Check sheet for the modelled part. Datum: model origin and axes. Units: mm. Face numbers are marked on the shaded views. A direction names the side the tool comes from. Round coordinates to 2 decimals unless told otherwise and drop trailing zeros. Write each loop counter-clockwise with the first axis right and the second up, starting at its lowest first coordinate (ties: lowest second). Pieces come first, ordered by that corner, then holes. Notation, with made-up numbers: (32, 25) -> (49, 25) arc R21 cw to (49, 45) -> close; hole circle Ø7 at (66, -24.5). An arc over 180 degrees is marked (long way). One line per item, written item: value.
from build123d import *

# Parameters (mm, degrees)
SKETCH_1_W          = 30
SKETCH_1_H          = 3
EXTRUDE_1_DEPTH     = 45
SKETCH_1_3_W        = 7
SKETCH_1_3_H        = 20
SKETCH_1_3_W_2      = 30
SKETCH_1_3_H_2      = 3
EXTRUDE_2_DEPTH     = 3
SKETCH_2_W          = 55
SKETCH_2_H          = 40
EXTRUDE_3_DEPTH     = 2
SKETCH_3_W          = 30
SKETCH_3_H          = 2
EXTRUDE_4_DEPTH     = 5
SKETCH_4_W          = 30
SKETCH_4_H          = 15
CUT_EXTRUDE_1_DEPTH = 58.203583804
CUT_EXTRUDE_2_REACH = 60.824
SKETCH_6_R          = 1.6
FILLET_1_R          = 3
FILLET_2_R          = 3
CHAMFER_1_SIZE      = 3
CHAMFER_2_SIZE      = 1
FILLET_4_R          = 3


# Some blends are built 0.0001 mm under size
with BuildPart() as part:
    # 草图1 → 凸台-拉伸1 (new body)
    with BuildSketch(Plane(origin=(0, 0, 0), x_dir=(1, 0, 0), z_dir=(0, 1, 0))):
        Polygon((18, 10), (15, 10), (15, 7), (15, -10), (18, -10), align=None)
        with Locations((0, 8.5)):
            Rectangle(SKETCH_1_W, SKETCH_1_H)
        Polygon((-15, 7), (-15, 10), (-18, 10), (-18, -10), (-15, -10), align=None)
    extrude(amount=-EXTRUDE_1_DEPTH)

    # 草图1<3> → 凸台-拉伸2 (add)
    with BuildSketch(Plane(origin=(0, 0, 0), x_dir=(1, 0, 0), z_dir=(0, 1, 0))):
        with Locations((-21.5, 0)):
            Rectangle(SKETCH_1_3_W, SKETCH_1_3_H)
        Polygon((-15, 7), (-15, 10), (-18, 10), (-18, -10), (-15, -10), align=None)
        with Locations((0, 8.5)):
            Rectangle(SKETCH_1_3_W_2, SKETCH_1_3_H_2)
        Polygon((18, 10), (15, 10), (15, 7), (15, -10), (18, -10), align=None)
        with Locations((21.5, 0)):
            Rectangle(SKETCH_1_3_W, SKETCH_1_3_H)
    extrude(amount=EXTRUDE_2_DEPTH)

    # 草图2 → 凸台-拉伸3 (add)
    with BuildSketch(Plane.XZ.offset(45)):
        Rectangle(SKETCH_2_W, SKETCH_2_H)
    extrude(amount=-EXTRUDE_3_DEPTH)

    # 草图3 → 凸台-拉伸4 (add)
    with BuildSketch(Plane(origin=(0, -43, 0), x_dir=(1, 0, 0), z_dir=(0, 1, 0))):
        with Locations((0, -9)):
            Rectangle(SKETCH_3_W, SKETCH_3_H)
    extrude(amount=EXTRUDE_4_DEPTH)

    # 草图4 → 切除-拉伸1 (cut, through all)
    with BuildSketch(Plane(origin=(0, -43, 0), x_dir=(1, 0, 0), z_dir=(0, 1, 0))):
        with Locations((0, -0.5)):
            Rectangle(SKETCH_4_W, SKETCH_4_H)
    extrude(amount=-CUT_EXTRUDE_1_DEPTH, mode=Mode.SUBTRACT)

    # 草图6 → 切除-拉伸2 (cut, up to next)
    with BuildSketch(Plane(origin=(0, 3, 0), x_dir=(1, 0, 0), z_dir=(0, 1, 0)), mode=Mode.PRIVATE) as cut_extrude_2_sk1:
        with Locations(Location((-22, -7, 0), (0, 0, 270))):
            Circle(SKETCH_6_R)
    cut_extrude_2_tool1 = extrude(cut_extrude_2_sk1.sketch, amount=-CUT_EXTRUDE_2_REACH, mode=Mode.PRIVATE) & part.part
    # 草图6 → 切除-拉伸2 (cut, up to next)
    with BuildSketch(Plane(origin=(0, 3, 0), x_dir=(1, 0, 0), z_dir=(0, 1, 0)), mode=Mode.PRIVATE) as cut_extrude_2_sk2:
        with Locations(Location((-22, 7, 0), (0, 0, 270))):
            Circle(SKETCH_6_R)
    cut_extrude_2_tool2 = extrude(cut_extrude_2_sk2.sketch, amount=-CUT_EXTRUDE_2_REACH, mode=Mode.PRIVATE) & part.part
    # 草图6 → 切除-拉伸2 (cut, up to next)
    with BuildSketch(Plane(origin=(0, 3, 0), x_dir=(1, 0, 0), z_dir=(0, 1, 0)), mode=Mode.PRIVATE) as cut_extrude_2_sk3:
        with Locations(Location((22, -7, 0), (0, 0, 270))):
            Circle(SKETCH_6_R)
    cut_extrude_2_tool3 = extrude(cut_extrude_2_sk3.sketch, amount=-CUT_EXTRUDE_2_REACH, mode=Mode.PRIVATE) & part.part
    # 草图6 → 切除-拉伸2 (cut, up to next)
    with BuildSketch(Plane(origin=(0, 3, 0), x_dir=(1, 0, 0), z_dir=(0, 1, 0)), mode=Mode.PRIVATE) as cut_extrude_2_sk4:
        with Locations(Location((22, 7, 0), (0, 0, 270))):
            Circle(SKETCH_6_R)
    cut_extrude_2_tool4 = extrude(cut_extrude_2_sk4.sketch, amount=-CUT_EXTRUDE_2_REACH, mode=Mode.PRIVATE) & part.part
    add(cut_extrude_2_tool1.solids().sort_by_distance((-22, 3, 7))[0], mode=Mode.SUBTRACT)
    add(cut_extrude_2_tool2.solids().sort_by_distance((-22, 3, -7))[0], mode=Mode.SUBTRACT)
    add(cut_extrude_2_tool3.solids().sort_by_distance((22, 3, 7))[0], mode=Mode.SUBTRACT)
    add(cut_extrude_2_tool4.solids().sort_by_distance((22, 3, -7))[0], mode=Mode.SUBTRACT)

    # 圆角1
    fillet_1_edges = [part.edges().sort_by_distance(p)[0] for p in [
        (-25, 1.5, 10),
        (25, 1.5, 10),
        (25, 1.5, -10),
        (-25, 1.5, -10),
    ]]
    fillet(fillet_1_edges, radius=FILLET_1_R)

    # 圆角2
    fillet_2_edges = [part.edges().sort_by_distance(p)[0] for p in [
        (-18, -21.5, -10),
        (18, -21.5, -10),
        (-18, -21.5, 10),
        (18, -21.5, 10),
        (27.5, -44, 20),
        (27.5, -44, -20),
        (-27.5, -44, -20),
        (-27.5, -44, 20),
    ]]
    fillet(fillet_2_edges, radius=FILLET_2_R - 0.0001)  # a hair under: the kernel refuses the full size

    # 倒角1
    chamfer_1_edges = [part.edges().sort_by_distance(p)[0] for p in [
        (0, -43, 10),
        (-18, -43, 0),
        (0, -43, -10),
        (18, -43, 0),
        (17.121349633, -43, 9.121349633),
        (-17.121349633, -43, 9.121349633),
        (17.121349633, -43, -9.121349633),
        (-17.121349633, -43, -9.121349633),
    ]]
    chamfer(chamfer_1_edges, length=CHAMFER_1_SIZE)

    # 倒角2
    # the kernel refuses this chamfer: 1 mm, written as the material it adds along each edge
    with BuildSketch(Plane(origin=(18, 0, 7.0001), x_dir=(0.9996219169112968, 0.027495876610586247, 0), z_dir=(0, 0, -1)), Plane(origin=(-18, 0, -7.0001), x_dir=(-0.9996219169112968, 0.02749587661058639, 0), z_dir=(0, 0, 1))) as chamfer_2_piece_1:
        Polygon((CHAMFER_2_SIZE * 0.999621916911, CHAMFER_2_SIZE * 0.0274958766106), (-CHAMFER_2_SIZE * 0.0274958766106, CHAMFER_2_SIZE * 0.999621916911), (0, 0), align=None)
    extrude(amount=14.0002)
    with BuildSketch(Plane(origin=(15.0001, 0, 7.0001), x_dir=(1, 0, 0), z_dir=(0, 0, -1))) as chamfer_2_piece_2_section:
        Polygon((2.9999 + CHAMFER_2_SIZE, 0), (2.9999, CHAMFER_2_SIZE), (2.9999, 0), align=None)
    chamfer_2_piece_2 = revolve(axis=Axis((15.0001, 0, 7.0001), (0, -1, 0)), revolution_arc=139.136895156, mode=Mode.PRIVATE)
    chamfer_2_piece_2 = split(chamfer_2_piece_2, bisect_by=Plane(origin=(18.290229606, -0.281148304, 10), z_dir=(0, 0, -1)), keep=Keep.TOP, mode=Mode.PRIVATE)
    chamfer_2_piece_2 = split(chamfer_2_piece_2, bisect_by=Plane(origin=(15, -0.281148304, 7.827153976), z_dir=(1, 0, 0)), keep=Keep.TOP, mode=Mode.PRIVATE)
    add(chamfer_2_piece_2)
    with BuildSketch(Plane(origin=(-15.0001, 0, 7.0001), x_dir=(-1, 0, 0), z_dir=(0, 0, -1))) as chamfer_2_piece_3_section:
        Polygon((2.9999 + CHAMFER_2_SIZE, 0), (2.9999, -CHAMFER_2_SIZE), (2.9999, 0), align=None)
    chamfer_2_piece_3 = revolve(axis=Axis((-15.0001, 0, 7.0001), (0, 1, 0)), revolution_arc=139.136895156, mode=Mode.PRIVATE)
    chamfer_2_piece_3 = split(chamfer_2_piece_3, bisect_by=Plane(origin=(-18.290229606, -0.281148304, 10), z_dir=(0, 0, -1)), keep=Keep.TOP, mode=Mode.PRIVATE)
    chamfer_2_piece_3 = split(chamfer_2_piece_3, bisect_by=Plane(origin=(-15, -0.281148304, 7.827153976), z_dir=(-1, 0, 0)), keep=Keep.TOP, mode=Mode.PRIVATE)
    add(chamfer_2_piece_3)
    with BuildSketch(Plane(origin=(15.0001, 0, -7.0001), x_dir=(-0.7562749275069748, 0, -0.6542539522420326), z_dir=(-0.6542539522420326, 0, 0.7562749275069748))) as chamfer_2_piece_4_section:
        Polygon((2.9999, CHAMFER_2_SIZE), (2.9999 + CHAMFER_2_SIZE, 0), (2.9999, 0), align=None)
    chamfer_2_piece_4 = revolve(axis=Axis((15.0001, 0, -7.0001), (0, -1, 0)), revolution_arc=139.136895156, mode=Mode.PRIVATE)
    chamfer_2_piece_4 = split(chamfer_2_piece_4, bisect_by=Plane(origin=(17.219196031, -0.376233932, -10), z_dir=(0, 0, 1)), keep=Keep.TOP, mode=Mode.PRIVATE)
    add(chamfer_2_piece_4)
    with BuildSketch(Plane(origin=(-15.0001, 0, -7.0001), x_dir=(0.7562749275069739, 0, -0.6542539522420336), z_dir=(0.6542539522420336, 0, 0.7562749275069739))) as chamfer_2_piece_5_section:
        Polygon((2.9999, -CHAMFER_2_SIZE), (2.9999 + CHAMFER_2_SIZE, 0), (2.9999, 0), align=None)
    chamfer_2_piece_5 = revolve(axis=Axis((-15.0001, 0, -7.0001), (0, 1, 0)), revolution_arc=139.136895156, mode=Mode.PRIVATE)
    chamfer_2_piece_5 = split(chamfer_2_piece_5, bisect_by=Plane(origin=(-17.219196031, -0.376233932, -10), z_dir=(0, 0, 1)), keep=Keep.TOP, mode=Mode.PRIVATE)
    add(chamfer_2_piece_5)

    # 圆角4
    fillet_4_edges = [part.edges().sort_by_distance(p)[0] for p in [
        (-15, -21, -7),
        (15, -21, -7),
        (-15, -41.5, 8),
        (15, -41.5, 8),
    ]]
    fillet(fillet_4_edges, radius=FILLET_4_R)


solid = part.part
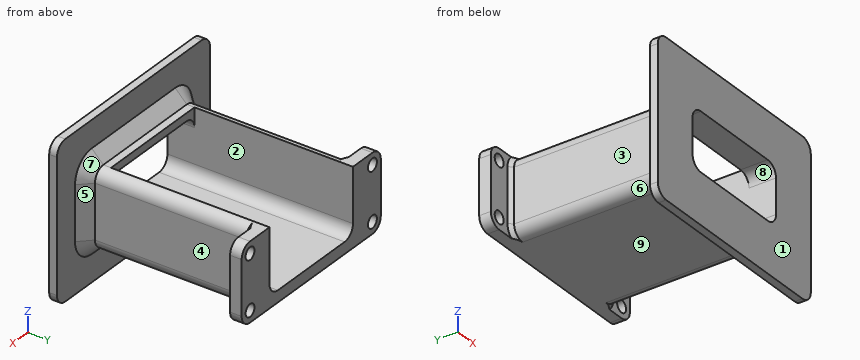
Item 1: Depth check by flat-ended pin: pin 1 (4 mm diameter, centred on x = 3.5, z = 8, fed in from +Y); pin 2 (4 mm diameter, centred on y = -29.5, z = -2.5, fed in from +X); pin 3 (7 mm diameter, centred on x = 0, y = -33, fed in from +Z). Enter the tip coordinate at first touch or a pass-through.
Result set:
pin 1: y = -38
pin 2: x = 18
pin 3: z = -7
Item 2: Tool access check on the marked faces 5, 6, 7, 8 and 9. Record the directions out of +Z, -Z, +X, -X, +Y, -Y that give a thin tool (end or side, any length) a straight path to the whole face; none if there is none.
Result set:
face 5: +Z, -Z, +X
face 6: -Z, -X
face 7: +Z, +X
face 8: +Y, -Y
face 9: -Z, +X, -X, +Y
Item 3: Sectioned sample at D-D (x = -13.5). Enter the section's corners in (y, z).
Result set:
outline: (-45, -20) -> (-43, -20) -> (-43, -13) -> (-40, -10) -> (3, -10) -> (3, -6.6) -> (-45, -6.6) -> close; (-45, 7.6) -> (-38, 7.6) -> (-38, 10) -> (-40, 10) -> (-43, 13) -> (-43, 20) -> (-45, 20) -> close
Item 4: Release check for a two-part mould opening along X. For the marked faces 1, 2, 3 and 4 record: pulls with the +X half, pulls with the -X half, needs draft (parallel to the pull), parting line crosses it, or undercut.
Result set:
face 1: needs draft
face 2: undercut
face 3: pulls with the -X half
face 4: pulls with the +X half
Item 5: Sectioned sample at A-A (x = 4). Enter the section's corners in (y, z), then the cut area to 3 significant figures.
Result set:
outline: (-45, -20) -> (-43, -20) -> (-43, -13) -> (-40, -10) -> (3, -10) -> (3, -7) -> (-45, -7) -> close; (-45, 8) -> (-38, 8) -> (-38, 10) -> (-40, 10) -> (-43, 13) -> (-43, 20) -> (-45, 20) -> close
area: 207 mm^2
Item 6: Material ranges on line 1 along X through (y, z) = (2.05, 7); line 2 along X through (y, z) = (-4, 1); line 3 along Y through (x, z) = (9, 9), recorded low to high.
Result set:
line 1: -25 to -23.6, -20.4 to -15, 15 to 20.4, 23.6 to 25
line 2: -18 to -15, 15 to 18
line 3: -45 to -38
Item 7: Sectioned sample at C-C (z = 14). Enter the section's corners in (x, y).
Result set:
outline: (-27.5, -45) -> (27.5, -45) -> (27.5, -43) -> (-27.5, -43) -> close
